The listing builds one solid part. Answer for the finished solid, in the listing's coordinates (mm). A direction names the side the tool comes from. Round coordinates to 2 decimals unless told otherwise and drop trailing zeros. Write each loop counter-clockwise with the first axis right and the second up, starting at its lowest first coordinate (ties: lowest second). Pieces come first, ordered by that corner, then holes. Notation, with made-up numbers: M 20,-27 L 43,-27 A4 ccw 43,-23 Z; hole C 52,17 d8. An arc over 180 degrees is marked long. One line per item, written item: value. Start each with the question number.
(1) Section A-A (x = -12) is taken. Determine the outline of the cut face in (y, z).
(2) Section B-B (z = 7.5) is taken. Determine the outline of the cut face in (x, y).
(3) Consider probe 1 along Y at (x, z) = (-19.5, 8.5); probe 2 along X at (y, z) = (7, 3.5); probe 3 along Y at (x, z) = (-24.5, 10). Determine where each line is inside the solid, lowest interval first.
(4) Section C-C (y = -4.5) is taken. Determine the outline of the cut face in (x, z).
(5) For a pull along X with two mould halves and no side action, classify faces 1 (the flat face through (27.559, 0, 7)), 2 (the flat face through (0, 0, 15.113)), 3 (the flat face through (0, 11.748, 6)) as released by +X, released by -X, zero draft, split by the parting line, or undercut.
(6) Section D-D (x = 0.5) is taken. Determine the outline of the cut face in (y, z).
(7) Given P1, Ø1.8, axis at x = -22.5, y = 10.5, coming from the -Z side; P2, Ø4, axis at x = -2, y = -0.5, coming from the -Z side, each flat-ended and moving along its own axis, determine where each tip first touches the part or whether it passes through.
(8) For faces 4 (the flat face through (-2, -13, 0)), 5 (the flat face through (0, 0, 11.938)), 6 (the flat face through (0, 8.496, 14)), determine the directions among +Z, -Z, +X, -X, +Y, -Y from which every point of the face is accessible in a straight line to the end or side of a thin tool.
Autodesk Inventor part; units mm, degrees
ref_plane "Work Plane1" through (0, 0, 11.938) normal (0, 0, 1) x (1, 0, 0)
ref_plane "YZ Plane" through (0, 0, 0) normal (1, 0, 0) x (0, 1, 0)
ref_plane "XZ Plane" through (0, 0, 0) normal (0, 1, 0) x (-1, 0, 0)
sketch "Sketch1" plane through (0, 0, 0) normal (0, 0, 1) x (1, 0, 0)
  line L0 (-27.559, -14.2875) -> (27.559, -14.2875)
  line L1 (27.559, -14.2875) -> (27.559, 14.2875)
  line L2 (27.559, 14.2875) -> (-27.559, 14.2875)
  line L3 (-27.559, 14.2875) -> (-27.559, -14.2875)
  line L4 (-27.559, -14.2875) -> (27.559, 14.2875) construction
  line L5 (27.559, -14.2875) -> (-27.559, 14.2875) construction
  line L6 (0, 0) -> (0, 51.7616) construction
  line L7 (-6.223, 8.4963) -> (6.223, 8.4963)
  line L8 (6.223, 8.4963) -> (6.223, 10.9347)
  line L9 (6.223, 10.9347) -> (-6.223, 10.9347)
  line L10 (-6.223, 10.9347) -> (-6.223, 8.4963)
  line L11 (-6.223, 8.4963) -> (6.223, 10.9347) construction
  line L12 (6.223, 8.4963) -> (-6.223, 10.9347) construction
  circle A0 centre (-23.241, 9.7155) radius 1.0795
  circle A1 centre (23.241, 9.7155) radius 1.0795
  circle A2 centre (-23.241, -9.7155) radius 1.0795
  circle A3 centre (23.241, -9.7155) radius 1.0795
  point P0 (0, 9.7155)
  dimension "d0" = 55.118
  dimension "d1" = 28.575
  dimension "d2" = 12.446
  dimension "d3" = 2.4384
  dimension "d11" = 4.572
  dimension "d12" = 2.159
  dimension "d13" = 2.159
  dimension "d14" = 4.318
  dimension "d15" = 4.318
  dimension "d16" = 2.159
  dimension "d17" = 4.572
  dimension "d18" = 2.159
ref_plane "Work Plane1" through (0, 0, 11.938) normal (0, 0, 1) x (1, 0, 0)
sketch "Sketch2" plane through (0, 0, 11.938) normal (0, 0, 1) x (1, 0, 0)
  line L0 (-25.019, -11.7475) -> (25.019, -11.7475)
  line L1 (25.019, -11.7475) -> (25.019, 11.7475)
  line L2 (25.019, 11.7475) -> (-25.019, 11.7475)
  line L3 (-25.019, 11.7475) -> (-25.019, -11.7475)
  line L4 (-25.019, -11.7475) -> (25.019, 11.7475) construction
  line L5 (25.019, -11.7475) -> (-25.019, 11.7475) construction
  line L6 (27.559, 14.2875) -> (-27.559, 14.2875)
  line L7 (-27.559, 14.2875) -> (-27.559, -14.2875)
  point P0 (0, 0)
  dimension "d7" = 2.54
  dimension "d8" = 2.54
extrude "Extrusion3" add sketch "Sketch1" along normal blind 15.113
ref_plane "Work Plane2" through (0, 0, 2.54) normal (0, 0, 1) x (1, 0, 0)
extrude "Extrusion6" cut sketch "Sketch2" against normal blind 12.573
sketch "Sketch4" plane through (0, 0, 11.938) normal (0, 0, -1) x (-1, 0, 0)
  circle A0 centre (-23.241, 9.7155) radius 1.0795
  circle A1 centre (-23.241, 9.7155) radius 1.0795
  circle A2 centre (-23.241, 9.7155) radius 1.778
  line L0 (-25.019, -11.7475) -> (-25.019, 11.7475)
  circle A3 centre (23.241, 9.7155) radius 1.0795
  circle A4 centre (23.241, 9.7155) radius 1.0795
  circle A5 centre (23.241, 9.7155) radius 1.778
  line L1 (25.019, 11.7475) -> (25.019, -11.7475)
  circle A6 centre (23.241, -9.7155) radius 1.0795
  circle A7 centre (23.241, -9.7155) radius 1.0795
  circle A8 centre (23.241, -9.7155) radius 1.778
  circle A9 centre (-23.241, -9.7155) radius 1.0795
  circle A10 centre (-23.241, -9.7155) radius 1.0795
  circle A11 centre (-23.241, -9.7155) radius 1.778
  point P0 (0, 0)
extrude "Extrusion7" add sketch "Sketch4" along normal blind 3.175
properties part number "Display"
Recorded:
1. outline: M -14.29,0 L -11.75,0 L -11.75,11.94 L 11.75,11.94 L 11.75,0 L 14.29,0 L 14.29,15.11 L -14.29,15.11 Z
2. outline: M -27.56,-14.29 L 27.56,-14.29 L 27.56,14.29 L -27.56,14.29 Z; hole M -25.02,-11.75 L 25.02,-11.75 L 25.02,11.75 L -25.02,11.75 Z
3. probe 1: y = -14.29 to -11.75, 11.75 to 14.29
3. probe 2: x = -27.56 to -25.02, 25.02 to 27.56
3. probe 3: y = -14.29 to -11.75, -10.97 to -8.46, 8.46 to 10.97, 11.75 to 14.29
4. outline: M -27.56,0 L -25.02,0 L -25.02,11.94 L 25.02,11.94 L 25.02,0 L 27.56,0 L 27.56,15.11 L -27.56,15.11 Z
5. face 1: released by +X
5. face 2: zero draft
5. face 3: undercut
6. outline: M -14.29,0 L -11.75,0 L -11.75,11.94 L 8.5,11.94 L 8.5,15.11 L -14.29,15.11 Z; M 10.93,11.94 L 11.75,11.94 L 11.75,0 L 14.29,0 L 14.29,15.11 L 10.93,15.11 Z
7. P1: stops at z = 8.76
7. P2: stops at z = 11.94
8. face 4: -Z, +X, -X, +Y, -Y
8. face 5: -Z
8. face 6: +Z, -Z
